Could you check a few things on this model? Use its own coordinates, in mm. A direction names the side the tool comes from. Coordinates: 2 decimals unless noted, no trailing zeros. Write each loop counter-clockwise with the first axis right and the second up, starting at its lowest first coordinate (ties: lowest second). Pieces come first, ordered by that corner, then holes.
Item 1: Thinking about a two-plate mould opening in X: for faces 4 (the cylindrical face through (0.477, -32.852, 2.809)), 5 (the flat face through (0, 42.5, 2)), 6 (the cylindrical face through (-2.1, -0.66, 2.81)), 7 (the flat face through (-4.4, -1, 2)), which applies, +X half, -X half, draft (parallel to the pull), parting line (faces both ways), or undercut?
Item 2: Which directions (+Z, -Z, +X, -X, +Y, -Y) give clear straight access to the entire face, cutting with the end or side of a thin tool? Please do faces 1 (the flat face through (6.65, -1, 0)), 2 (the flat face through (-6, -1, 0.85)), 3 (the flat face through (6, -1, 0.85)).
Item 3: I want a section at C-C on y = -13.5. Please give me the cut outline in (x, z), then the cut area to 4 significant figures.
Item 4: If I drill on probe 1 along Y at (x, z) = (0, 2); probe 2 along X at (y, z) = (35, 3.4); probe 3 along X at (y, z) = (-2, 0.65), over which ranges is the centre line in solid material (lowest first)?
Item 5: For P1, Ø1, axis at y = 12, z = 3, coming from the -X side; P2, Ø1.8, axis at x = 5.5, y = -6.5, coming from the +Z side; P3, Ø5.5, axis at x = 0, y = 35, coming from the -Z side; P4, Ø2.5, axis at x = -5.5, y = 10.5, coming from the +Z side, each with a flat end and sliding along its axis, tell me the tip position at first contact or that it passes through.
Item 6: I want a section at A-A on z = 0.1. Please give me the cut outline in (x, y).
Item 7: I want a section at B-B on y = 35. Please give me the cut outline in (x, z), then the cut area to 3 significant figures.
from build123d import *

# Parameters (mm, degrees)
F0_W           = 8.8
F0_H           = 3.3
F1_DEPTH       = 42.5
F3_D           = 4.4
F3_CSINK_D     = 8.96
F3_CSINK_ANGLE = 90


with BuildPart() as f1:
    # F0 (on Front) → F1 (new body, symmetric)
    with BuildSketch(Plane.XZ):
        Polygon((6.65, -0.85), (6.65, 0.85), (4.4, 0.85), (-4.4, 0.85), (-6.65, 0.85), (-6.65, -0.85), align=None)
        with Locations((0, 2.5)):
            Rectangle(F0_W, F0_H)
    extrude(amount=F1_DEPTH, both=True)

    # F3 (through all)
    with Locations(Plane(origin=(0, 0, -0.85), x_dir=(1, 0, 0), z_dir=(0, 0, -1))):
        with Locations((0, -35), (0, 0), (0, 35)):
            CounterSinkHole(F3_D / 2, F3_CSINK_D / 2, counter_sink_angle=F3_CSINK_ANGLE)


solid = f1.part
Response values:
1. face 4: undercut
1. face 5: draft
1. face 6: undercut
1. face 7: -X half
2. face 1: +Z, -Z, +X, +Y, -Y
2. face 2: +Z, -X, +Y, -Y
2. face 3: +Z, +X, +Y, -Y
3. outline: (-6.65, -0.85) - (6.65, -0.85) - (6.65, 0.85) - (4.4, 0.85) - (4.4, 4.15) - (-4.4, 4.15) - (-4.4, 0.85) - (-6.65, 0.85) - close
3. area: 51.65 mm2
4. probe 1: y = -42.5 to -37.2, -32.8 to -2.2, 2.2 to 32.8, 37.2 to 42.5
4. probe 2: x = -4.4 to -2.2, 2.2 to 4.4
4. probe 3: x = -6.65 to -2.21, 2.21 to 6.65
5. P1: stops at x = -4.4
5. P2: stops at z = 0.85
5. P3: stops at z = 0.88
5. P4: stops at z = 4.15
6. outline: (-6.65, -42.5) - (6.65, -42.5) - (6.65, 42.5) - (-6.65, 42.5) - close; hole circle Ø7.06 at (0, -35); hole circle Ø7.06 at (0, 0); hole circle Ø7.06 at (0, 35)
7. outline: (-6.65, -0.85) - (-4.48, -0.85) - (-2.2, 1.43) - (-2.2, 4.15) - (-4.4, 4.15) - (-4.4, 0.85) - (-6.65, 0.85) - close; (2.2, 1.43) - (4.48, -0.85) - (6.65, -0.85) - (6.65, 0.85) - (4.4, 0.85) - (4.4, 4.15) - (2.2, 4.15) - close
7. area: 24.5 mm2
